```python
from build123d import *

# Parameters (mm, degrees)
BOX002_W     = 4
BOX002_H     = 7
BOX002_DEPTH = 1
BOX007_W     = 4
BOX007_H     = 2
BOX007_DEPTH = 5.3
BOX003_W     = 4
BOX003_H     = 2
BOX003_DEPTH = 5.3


with BuildPart() as cubo003:
    # Box002 → Box002 (new body)
    with BuildSketch(Plane(origin=(0, 1, 0), x_dir=(1, 0, 0), z_dir=(0, 0, 1))):
        with Locations((2, 3.5)):
            Rectangle(BOX002_W, BOX002_H)
    extrude(amount=BOX002_DEPTH)


with BuildPart() as cubo006:
    # Box007 → Box007 (new body)
    with BuildSketch(Plane(origin=(0, 8, 0), x_dir=(1, 0, 0), z_dir=(0, 0, 1))):
        with Locations((2, 1)):
            Rectangle(BOX007_W, BOX007_H)
    extrude(amount=BOX007_DEPTH)


with BuildPart() as bridge:
    # Box003 → Box003 (new body)
    with BuildSketch(Plane(origin=(0, -1, 0), x_dir=(1, 0, 0), z_dir=(0, 0, 1))):
        with Locations((2, 1)):
            Rectangle(BOX003_W, BOX003_H)
    extrude(amount=BOX003_DEPTH)

    # Fusion007: union Cubo003, Cubo006
    add(cubo003.part)
    add(cubo006.part)


with BuildPart() as bridge_1:
    # Fusion007 placement: moved
    add(bridge.part.moved(Location((-9, -4.5, 91.81))))


solid = bridge_1.part
```
Here's how the part is built. I have some questions about the finished solid (model axes, mm). A direction names the side the tool comes from. Round coordinates to 2 decimals unless told otherwise and drop trailing zeros. Order: outer loops, then holes, each group sorted by start corner. A loop starts at its lowest first (then second) coordinate and runs counter-clockwise, first axis right, second up. Notation, with made-up numbers: M -10.5,-28 L 25.5,-28 A18 cw 25.5,-6 Z; hole C 6.5,-20.5 d10. An arc over 180 degrees is marked long. One line per question, with ' | ' between items.
1) If we mould it in two halves opening along Y, with no side actions, what happens to faces 3 (the face through (-7, 3.5, 95)), 4 (the face through (-7, 0, 91.81)), 5 (the face through (-7, 5.5, 94)), 6 (the face through (-7, 0, 92.81))? For each: +Y half, -Y half, draft (parallel to the pull), parting line (faces both ways), or undercut.
Working result:
face 3: undercut | face 4: draft | face 5: +Y half | face 6: undercut
2) I want a section at A-A, the plane z = 95.4. Write out the boundary of the cut face in (x, y).
Working result:
outline: M -9,-5.5 L -5,-5.5 L -5,-3.5 L -9,-3.5 Z; M -9,3.5 L -5,3.5 L -5,5.5 L -9,5.5 Z
3) For pin 1 Ø2 at (x, y) = (-6.5, -1) entering from +Z, with a flat end and sliding along its axis, tell me the tip position at first contact or that it passes through.
Working result:
pin 1: z = 92.81
4) I want a section at C-C, the plane y = 3. Write out the boundary of the cut face in (x, z).
Working result:
outline: M -9,91.81 L -5,91.81 L -5,92.81 L -9,92.81 Z
5) For faces 1 (the face through (-9, -0.08, 92.66)), 2 (the face through (-7, -3.5, 95)), which set-ups out of +Z, -Z, +X, -X, +Y, -Y let a thin tool reach every point of the face, with its end or its side?
Working result:
face 1: +Z, -Z, -X, +Y, -Y | face 2: +Z, +X, -X
6) I want a section at B-B, the plane x = -5.8. Write out the boundary of the cut face in (y, z).
Working result:
outline: M -5.5,91.81 L 5.5,91.81 L 5.5,97.11 L 3.5,97.11 L 3.5,92.81 L -3.5,92.81 L -3.5,97.11 L -5.5,97.11 Z
7) I need wall thicknesses on line 1 along Y through (x, z) = (-6.6, 93.9); line 2 along Z through (x, y) = (-7, 2.75). Which ranges of each line are inside material? Lowest first, please.
Working result:
line 1: -5.5 to -3.5, 3.5 to 5.5 | line 2: 91.81 to 92.81
